Check sheet for the drawn part. Datum: minimum x, y, z corner. Units: mm. Coordinates: 2 decimals unless noted, no trailing zeros. Order: outer loops, then holes, each group sorted by start corner. A loop starts at its lowest first (then second) coordinate and runs counter-clockwise, first axis right, second up.
Q1. Cross-section at A-A, the plane z = 76.2. Record the boundary of the cut face in (x, y), and give its area (3 significant figures).
Q2. Thickness scan on line 1 (Z direction, x = 196.85, y = 25.5); line 2 (X direction, y = 9, z = 88); line 3 (Z direction, x = 138, y = 11). Record the ranges inside material, lowest first.
Q3. Cross-section at D-D, the plane x = 145. Record the boundary of the cut face in (y, z), and give its area (3 significant figures).
Q4. Cross-section at B-B, the plane y = 30. Record the boundary of the cut face in (x, z), and give its area (3 significant figures).
Q5. Depth check by flat-ended pin: P1, Ø23, axis at x = 69.85, z = 76.2, coming from the -Y side. Enter the tip coordinate at first touch or a pass-through.
Q6. Cross-section at C-C, the plane x = 69.85. Record the boundary of the cut face in (y, z), and give its area (3 significant figures).
Q7. Draft check along Z on the marked faces 1, 2, 3 and 4. Enter one of: pulls with the +Z half, pulls with the -Z half, needs draft (parallel to the pull), parting line crosses it, or undercut.
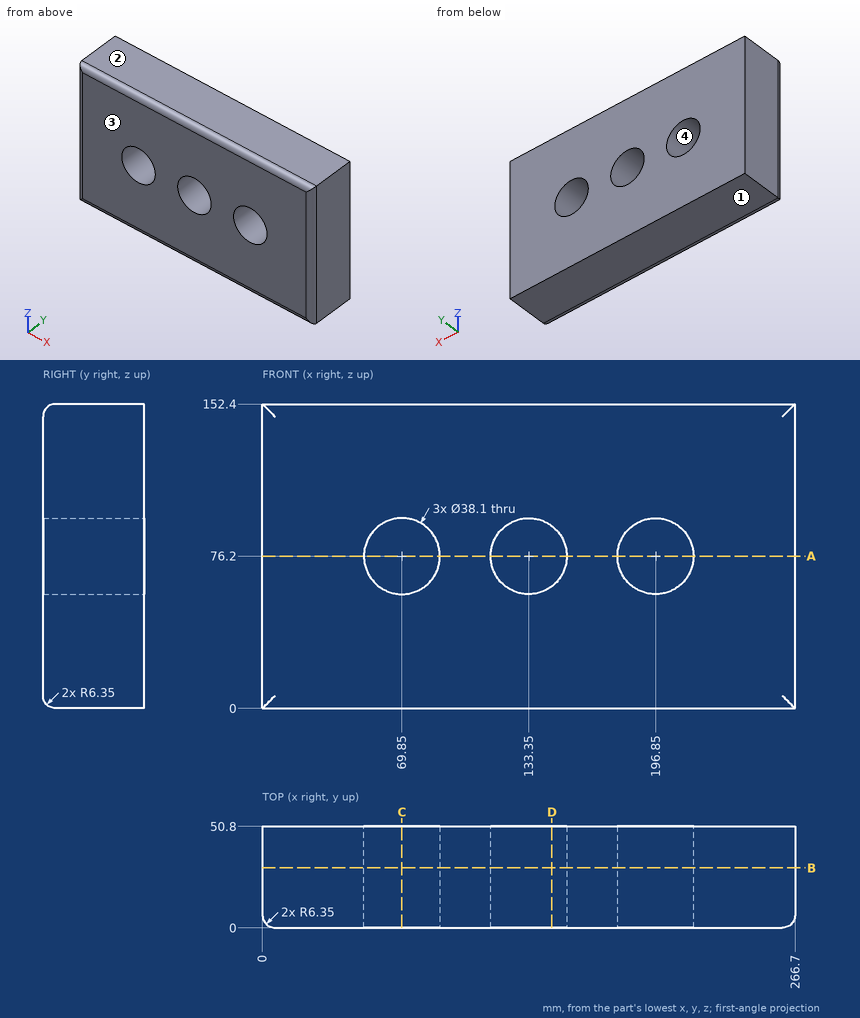
Check values:
1. outline: (0, 6.35) arc R6.35 ccw to (6.35, 0) - (50.8, 0) - (50.8, 50.8) - (0, 50.8) - close; (88.9, 0) - (114.3, 0) - (114.3, 50.8) - (88.9, 50.8) - close; (152.4, 0) - (177.8, 0) - (177.8, 50.8) - (152.4, 50.8) - close; (215.9, 0) - (260.35, 0) arc R6.35 ccw to (266.7, 6.35) - (266.7, 50.8) - (215.9, 50.8) - close
1. area: 7,720 mm2
2. line 1: z = 0 to 57.15, 95.25 to 152.4
2. line 2: x = 0 to 54.89, 84.81 to 118.39, 148.31 to 181.89, 211.81 to 266.7
2. line 3: z = 0 to 57.73, 94.67 to 152.4
3. outline: (0, 6.35) arc R6.35 ccw to (6.35, 0) - (50.8, 0) - (50.8, 61.13) - (0, 61.13) - close; (0, 91.27) - (50.8, 91.27) - (50.8, 152.4) - (6.35, 152.4) arc R6.35 ccw to (0, 146.05) - close
3. area: 6,190 mm2
4. outline: (0, 0) - (266.7, 0) - (266.7, 152.4) - (0, 152.4) - close; hole circle Ø38.1 at (69.85, 76.2); hole circle Ø38.1 at (133.35, 76.2); hole circle Ø38.1 at (196.85, 76.2)
4. area: 37,200 mm2
5. P1: passes through
6. outline: (0, 6.35) arc R6.35 ccw to (6.35, 0) - (50.8, 0) - (50.8, 57.15) - (0, 57.15) - close; (0, 95.25) - (50.8, 95.25) - (50.8, 152.4) - (6.35, 152.4) arc R6.35 ccw to (0, 146.05) - close
6. area: 5,790 mm2
7. face 1: pulls with the -Z half
7. face 2: pulls with the +Z half
7. face 3: needs draft
7. face 4: undercut
